```python
from build123d import *

# Parameters (mm, degrees)
F0_W     = 254
F0_H     = 368.3
F1_DEPTH = 292.1
F2_R     = 35.73197
F3_DEPTH = 25.4
F4_R     = 10.16


with BuildPart() as f1:
    # F0 (on Front) → F1 (new body)
    with BuildSketch(Plane.XZ):
        with Locations((0.303643, -28.702023)):
            Rectangle(F0_W, F0_H)
    extrude(amount=F1_DEPTH)

    # F2 (on face) → F3 (join)
    with BuildSketch(Plane.XY.offset(155.447977)):
        with Locations((50.064862, -196.309745)):
            Circle(F2_R)
    extrude(amount=F3_DEPTH)

    # F4
    f4_edges = [f1.edges().sort_by_distance(p)[0] for p in [
        (-126.696357, -292.1, -28.702023),
        (0.303643, -292.1, 155.447977),
        (-126.696357, -146.05, 155.447977),
        (0.303643, 0, 155.447977),
        (127.303643, -146.05, 155.447977),
        (-126.696357, 0, -28.702023),
        (-126.696357, -146.05, -212.852023),
        (0.303643, 0, -212.852023),
        (127.303643, 0, -28.702023),
        (127.303643, -292.1, -28.702023),
        (0.303643, -292.1, -212.852023),
        (127.303643, -146.05, -212.852023),
    ]]
    fillet(f4_edges, radius=F4_R)


solid = f1.part
```
Input: part model. Units: mm. Frame: model coordinates. A direction names the side the tool comes from. Coordinates: 2 decimals unless noted, no trailing zeros. Write each loop counter-clockwise with the first axis right and the second up, starting at its lowest first coordinate (ties: lowest second). Pieces come first, ordered by that corner, then holes. Notation, with made-up numbers: (-27, 85) -> (-23, 85) arc R25 cw to (-23, 98) -> close; hole circle Ø8 at (49, 84.25). An arc over 180 degrees is marked (long way). Answer as a JSON object with one key per item and string values.
1. Section B-B on x = -81. Return the cut outline in (y, z).
Result set:
{"outline": "(-292.1, -202.69) arc R10.16 ccw to (-281.94, -212.85) -> (-10.16, -212.85) arc R10.16 ccw to (0, -202.69) -> (0, 145.29) arc R10.16 ccw to (-10.16, 155.45) -> (-281.94, 155.45) arc R10.16 ccw to (-292.1, 145.29) -> close"}
2. Section D-D on x = 46.5. Return the cut outline in (y, z), then the cut area to 3 significant figures.
Result set:
{"outline": "(-292.1, -202.69) arc R10.16 ccw to (-281.94, -212.85) -> (-10.16, -212.85) arc R10.16 ccw to (0, -202.69) -> (0, 145.29) arc R10.16 ccw to (-10.16, 155.45) -> (-160.76, 155.45) -> (-160.76, 180.85) -> (-231.86, 180.85) -> (-231.86, 155.45) -> (-281.94, 155.45) arc R10.16 ccw to (-292.1, 145.29) -> close", "area": "109,000 mm2"}
3. Section C-C on y = -177.5. Return the cut outline in (x, z), then the cut area to 3 significant figures.
Result set:
{"outline": "(-126.7, -202.69) arc R10.16 ccw to (-116.54, -212.85) -> (117.14, -212.85) arc R10.16 ccw to (127.3, -202.69) -> (127.3, 145.29) arc R10.16 ccw to (117.14, 155.45) -> (80.45, 155.45) -> (80.45, 180.85) -> (19.68, 180.85) -> (19.68, 155.45) -> (-116.54, 155.45) arc R10.16 ccw to (-126.7, 145.29) -> close", "area": "95,000 mm2"}
4. Material intervals for line 1 (Z direction, x = -78, y = -201); line 2 (Y direction, x = 70, z = 154), sorted ascending. Write a range as from..to.
Result set:
{"line 1": "z = -212.85..155.45", "line 2": "y = -287.17..-4.93"}
5. Section A-A on y = -32.5. Return the cut outline in (x, z).
Result set:
{"outline": "(-126.7, -202.69) arc R10.16 ccw to (-116.54, -212.85) -> (117.14, -212.85) arc R10.16 ccw to (127.3, -202.69) -> (127.3, 145.29) arc R10.16 ccw to (117.14, 155.45) -> (-116.54, 155.45) arc R10.16 ccw to (-126.7, 145.29) -> close"}
6. Access query for faces 1 (the face through (45.413, -160.882, 167.97)), 2 (the face through (1.939, -3.055, 152.551)). Directions: +Z, -Z, +X, -X, +Y, -Y. A direction counts if a zero-diameter tool reaches every point of the face in a straight line with its end or side. Return the directions, or none.
Result set:
{"face 1": "+Z", "face 2": "+Z, +X, -X, +Y"}
